Job drawing, mm, ordinate dimensions from the low corner. One solid piece. A direction names the side the tool comes from. Round coordinates to 2 decimals unless told otherwise and drop trailing zeros. Loops run counter-clockwise (first coordinate to the right, second up) from the corner with the lowest first, then second, coordinate; pieces in that order, holes last.
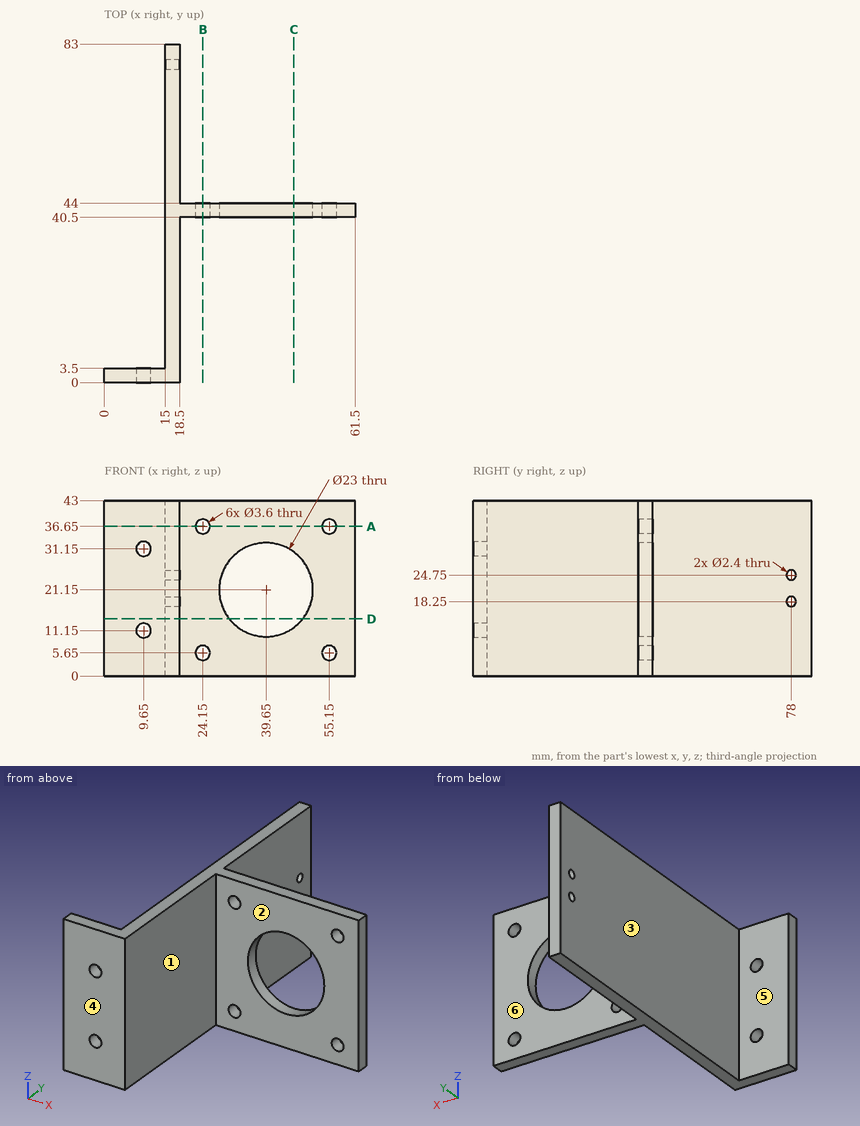
(1) Pull direction X, two halves, no side cores. Call the marked faces 1, 2 and 3: +X half, -X half, draft (parallel to the pull), parting line (faces both ways), or undercut.
Responses:
face 1: +X half
face 2: draft
face 3: -X half
(2) Slice it at C-C on x = 46.5. List the corners of the cut face in (y, z).
Responses:
outline: (40.5, 0) - (44, 0) - (44, 11.91) - (40.5, 11.91) - close; (40.5, 30.39) - (44, 30.39) - (44, 43) - (40.5, 43) - close
(3) Probe line 1 (Z direction, x = 55.15, y = 41.65); line 2 (X direction, y = 42, z = 5); line 3 (X direction, y = 42.5, z = 21). List the from-to ranges inside material, lowest first.
Responses:
line 1: z = 0 to 3.85, 7.45 to 34.85, 38.45 to 43
line 2: x = 15 to 22.47, 25.83 to 53.47, 56.83 to 61.5
line 3: x = 15 to 28.15, 51.15 to 61.5
(4) Which spindle directions (+Z, -Z, +X, -X, +Y, -Y) get a long thin tool onto all of the face, cutting with end or side? Do the marked faces 4, 5 and 6. Say none if no direction does.
Responses:
face 4: +Z, -Z, +X, -X, -Y
face 5: +Z, -Z, -X, +Y
face 6: +Z, -Z, +X, +Y
(5) Pin check, flat tips, straight feed: P1, Ø1.5, axis at x = 55, z = 13, coming from the +Y side; P2, Ø1, axis at y = 9, z = 8, coming from the -X side; P3, Ø16.5, axis at x = 8.5, z = 31, coming from the +Y side; P4, Ø2, axis at y = 10.5, z = 33.5, coming from the +X side. Stop position of each tip, or through.
Responses:
P1: stops at y = 44
P2: stops at x = 15
P3: stops at y = 83
P4: stops at x = 18.5
(6) Slice it at D-D on z = 14. List the corners of the cut face in (x, y).
Responses:
outline: (0, 0) - (18.5, 0) - (18.5, 40.5) - (30.64, 40.5) - (30.64, 44) - (18.5, 44) - (18.5, 83) - (15, 83) - (15, 3.5) - (0, 3.5) - close; (48.66, 40.5) - (61.5, 40.5) - (61.5, 44) - (48.66, 44) - close
(7) Slice it at A-A on z = 36.65. List the corners of the cut face in (x, y).
Responses:
outline: (0, 0) - (18.5, 0) - (18.5, 40.5) - (22.35, 40.5) - (22.35, 44) - (18.5, 44) - (18.5, 83) - (15, 83) - (15, 3.5) - (0, 3.5) - close; (25.95, 40.5) - (53.35, 40.5) - (53.35, 44) - (25.95, 44) - close; (56.95, 40.5) - (61.5, 40.5) - (61.5, 44) - (56.95, 44) - close
(8) Slice it at B-B on x = 24.15. List the corners of the cut face in (y, z).
Responses:
outline: (40.5, 0) - (44, 0) - (44, 3.85) - (40.5, 3.85) - close; (40.5, 7.45) - (44, 7.45) - (44, 34.85) - (40.5, 34.85) - close; (40.5, 38.45) - (44, 38.45) - (44, 43) - (40.5, 43) - close
